Geometry: see drawing. Coordinates: mm, zero at the bounding-box minimum. A direction names the side the tool comes from. Round coordinates to 2 decimals unless told otherwise and drop trailing zeros. Write each loop counter-clockwise with the first axis right and the second up, starting at its lowest first coordinate (ties: lowest second). Pieces come first, ordered by that corner, then holes. Notation, with made-up numbers: (-27.75, 59) -> (12.25, 59) arc R23 cw to (12.25, 71) -> close; hole circle Ø11 at (-28.5, 8.5). An arc over 180 degrees is marked (long way). Use CSV: the item, a comma, the result in double quotes.
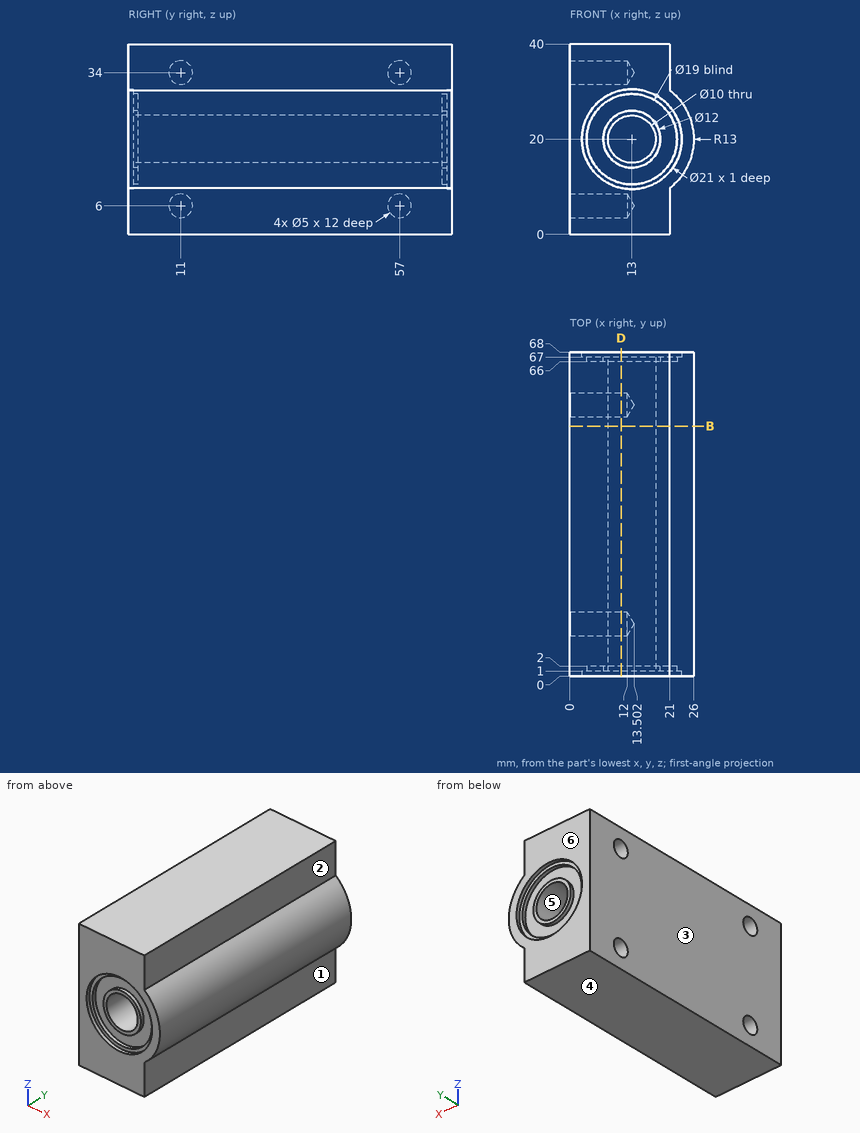
Item 1: First-contact query: pin 1 Ø3 at (y, z) = (57, 34) entering from -X; pin 2 Ø9.5 at (x, z) = (14.5, 18.5) entering from -Y; pin 3 Ø3 at (y, z) = (23, 35.5) entering from +X. Flat tips, straight axial feed; report the tip coordinate or a pass-through.
Worked answers:
pin 1,"stops at x = 12.6"
pin 2,"stops at y = 1"
pin 3,"stops at x = 21"
Item 2: Section query B-B on y = 52.5. Return the cut outline in (x, z).
Worked answers:
outline,"(0, 0) -> (21, 0) -> (21, 9.75) arc R13 ccw to (21, 30.25) -> (21, 40) -> (0, 40) -> close; hole circle Ø10 at (13, 20)"
Item 3: Set-up query: the marked faces 1, 2 and 3. Return all of +Z, -Z, +X, -X, +Y, -Y with unobstructed straight access to the full face (end or side cutting, diameter ignored); none if empty.
Worked answers:
face 1,"-Z, +X, +Y, -Y"
face 2,"+Z, +X, +Y, -Y"
face 3,"+Z, -Z, -X, +Y, -Y"
Item 4: Pull-direction query (Z, two-part tool) for the marked faces 4, 5 and 6; classes: +Z half, -Z half, draft (parallel to the pull), parting line (faces both ways), or undercut.
Worked answers:
face 4,"-Z half"
face 5,"undercut"
face 6,"draft"
Item 5: Line query: line 1 (Z direction, x = 13, y = 66.55); line 2 (Y direction, x = 6.25, z = 34); line 3 (Z direction, x = 2, y = 59). Output: solid intervals per line, ascending.
Worked answers:
line 1,"z = 0 to 10.5, 14 to 15, 25 to 26, 29.5 to 40"
line 2,"y = 0 to 8.5, 13.5 to 54.5, 59.5 to 68"
line 3,"z = 0 to 4.5, 7.5 to 32.5, 35.5 to 40"
Item 6: Section query D-D on x = 10.75. Give the number of separate pieces and of enclosed holes in the cut face, plus the area to 3 significant figures.
Worked answers:
separate pieces,"2"
enclosed holes,"4"
area,"2,000 mm²"
